Can you work these out from the model? Positions are in its coordinate system, mm. A direction names the side the tool comes from. Coordinates: 2 decimals unless noted, no trailing zeros. Loops run counter-clockwise (first coordinate to the right, second up) from the corner with the lowest first, then second, coordinate; pieces in that order, holes last. Notation, with made-up numbers: (72.25, -19.5) -> (113.25, -19.5) arc R35 ccw to (113.25, 14.5) -> close; hole circle Ø3 at (-21.5, 37.5). An arc over 180 degrees is marked (long way). Use one line per item in the form item = value. Start each with the question number.
(1) Imagine slicing it at A-A (x = 15). List the corners of the cut face in (y, z) for me, plus the area to 3 significant figures.
(2) On a 3-axis mill with a long thin cutter (end or side, diameter ignored), from which of +Z, -Z, +X, -X, +Y, -Y can I reach the whole of each face in a straight line? I mean faces 1 (the flat face through (-7.095, -3.109, -0.096)), 2 (the cylindrical face through (19.388, -5.224, 0.003)). Say none if no direction works.
(3) Imagine slicing it at B-B (y = -2.5). List the corners of the cut face in (x, z) for me, plus the area to 3 significant figures.
(4) I need wall thicknesses on line 1 (Y direction, x = 13.5, z = 0.05); line 2 (Y direction, x = 16.5, z = 0.1); line 3 (Y direction, x = 17.5, z = 0.1). Which ranges of each line are inside material? Lowest first, please. Write a range as [from, to].
(5) Thinking about a two-plate mould opening in X: for faces 3 (the flat face through (8, -1, 0.19)), 4 (the flat face through (21.98, -5.36, 0)), 5 (the cylindrical face through (17.016, -2.473, 0.003)), which applies, released by +X, released by -X, zero draft, split by the parting line, or undercut?
(6) Imagine slicing it at C-C (x = 3.5). List the corners of the cut face in (y, z) for me (3 decimals).
(7) Imagine slicing it at D-D (x = -12). List the corners of the cut face in (y, z) for me, plus the area to 3 significant figures.
```python
from build123d import *

# Parameters (mm, degrees)
BOSS_EXTRU_1_DEPTH           = 0.19
ENL_V_MAT_EXTRU_1_DEPTH      = 24.560167769
CONG_1_R                     = 0.25
ENL_V_MAT_EXTRU_2_DEPTH      = 21.94767488
ENL_V_MAT_EXTRU_2_DEPTH_BACK = 21.94767488


with BuildPart() as part:
    # Esquisse1 → Boss.-Extru.1 (new, symmetric)
    with BuildSketch(Plane.XY):
        with BuildLine():
            Line((-17.183394089, -0.900543525), (0, 0))
            Line((0, 0), (20, 0))
            Line((20, 0), (22.816605911, -4.878504542))
            Line((22.816605911, -4.878504542), (21.116605911, -5.86))
            ThreePointArc((21.116605911, -5.86), (19.362950472, -5.217969417), (17.508226773, -5))
            Line((17.508226773, -5), (4.724985048, -5))
            ThreePointArc((4.724985048, -5), (2.870261349, -5.217969417), (1.116605911, -5.86))
            Line((1.116605911, -5.86), (-17.183394089, -0.900543525))
        make_face()
    extrude(amount=BOSS_EXTRU_1_DEPTH, both=True)

    # Esquisse2 → Enlèv. mat.-Extru.1 (cut, through all)
    with BuildSketch(Plane.XY.offset(0.19)):
        with BuildLine():
            Line((-0.983394089, -1.85), (0.016605911, -1.85))
            Line((0.016605911, -1.85), (0.016605911, -1.675))
            Line((0.016605911, -1.675), (7.016605911, -1.675))
            Line((7.016605911, -1.675), (7.016605911, -1.25))
            Line((7.016605911, -1.25), (15.766605911, -1.25))
            ThreePointArc((15.766605911, -1.25), (17.016605911, -2.5), (15.766605911, -3.75))
            Line((15.766605911, -3.75), (7.016605911, -3.75))
            Line((7.016605911, -3.75), (7.016605911, -3.325))
            Line((7.016605911, -3.325), (0.016605911, -3.325))
            Line((0.016605911, -3.325), (0.016605911, -3.15))
            Line((0.016605911, -3.15), (-0.983394089, -3.15))
            Line((-0.983394089, -3.15), (-0.983394089, -1.85))
        make_face()
    extrude(amount=-ENL_V_MAT_EXTRU_1_DEPTH, mode=Mode.SUBTRACT)

    # Congé1
    # the kernel refuses this fillet: 0.25 mm, written as the material it adds along each edge
    with BuildSketch(Plane(origin=(7.016605911, -3.75, 0.19), x_dir=(0, 1, 0), z_dir=(0, 0, -1))) as cong_1_piece_1:
        with BuildLine():
            CenterArc((CONG_1_R, CONG_1_R), CONG_1_R, 180, 90)
            Line((0, CONG_1_R), (-CONG_1_R * 0.02, CONG_1_R))
            Line((-CONG_1_R * 0.02, CONG_1_R), (-CONG_1_R * 0.02, -CONG_1_R * 0.02))
            Line((-CONG_1_R * 0.02, -CONG_1_R * 0.02), (CONG_1_R, -CONG_1_R * 0.02))
            Line((CONG_1_R, -CONG_1_R * 0.02), (CONG_1_R, 0))
        make_face()
    extrude(amount=0.38)
    with BuildSketch(Plane(origin=(7.016605911, -1.25, 0.19), x_dir=(0, -1, 0), z_dir=(0, 0, -1)), Plane(origin=(-0.983394089, -3.15, 0.19), x_dir=(1, 0, 0), z_dir=(0, 0, -1)), Plane(origin=(-0.983394089, -1.85, 0.19), x_dir=(0, -1, 0), z_dir=(0, 0, -1))) as cong_1_piece_2:
        with BuildLine():
            CenterArc((CONG_1_R, -CONG_1_R), CONG_1_R, 90, 90)
            Line((0, -CONG_1_R), (-CONG_1_R * 0.02, -CONG_1_R))
            Line((-CONG_1_R * 0.02, -CONG_1_R), (-CONG_1_R * 0.02, CONG_1_R * 0.02))
            Line((-CONG_1_R * 0.02, CONG_1_R * 0.02), (CONG_1_R, CONG_1_R * 0.02))
            Line((CONG_1_R, CONG_1_R * 0.02), (CONG_1_R, 0))
        make_face()
    extrude(amount=0.38)
    with BuildSketch(Plane(origin=(0.016605911, -3.325, 0.19), x_dir=(1, 0, 0), z_dir=(0, 0, -1))) as cong_1_piece_3:
        with BuildLine():
            CenterArc((0.2384848, -0.25), CONG_1_R, 90, 72.542396876)
            Line((0, -0.175), (-0.004769696, -0.1735))
            ThreePointArc((-0.004769696, -0.1735), (-0.005, -0.0875), (-0.005, 0))
            Line((-0.005, 0), (0, 0.005))
            Line((0, 0.005), (0.2384848, 0.005))
            Line((0.2384848, 0.005), (0.2384848, 0))
        make_face()
    extrude(amount=0.38)
    with BuildSketch(Plane(origin=(0.016605911, -1.675, 0.19), x_dir=(0, -1, 0), z_dir=(0, 0, -1))) as cong_1_piece_4:
        with BuildLine():
            CenterArc((0.25, -0.2384848), CONG_1_R, 107.457603124, 72.542396876)
            Line((0, -0.2384848), (-0.005, -0.2384848))
            Line((-0.005, -0.2384848), (-0.005, 0))
            Line((-0.005, 0), (0, 0.005))
            ThreePointArc((0, 0.005), (0.0875, 0.005), (0.1735, 0.004769696))
            Line((0.1735, 0.004769696), (0.175, 0))
        make_face()
    extrude(amount=0.38)

    # Esquisse3 → Enlèv. mat.-Extru.2 (cut, two sides: drawn at the far end of the back side and taken through both)
    with BuildSketch(Plane(origin=(2.519658127, -0.682848897, 0), x_dir=(0, 0, 1), z_dir=(-0.9651836866427717, 0.26157303194073345, 0)).offset(-ENL_V_MAT_EXTRU_2_DEPTH_BACK)):
        Polygon((0, -5.36390241), (0.19, -4.36390241), (0.19, -5.53890241), (-0.19, -5.53890241), (-0.19, -4.36390241), align=None)
    extrude(amount=ENL_V_MAT_EXTRU_2_DEPTH + ENL_V_MAT_EXTRU_2_DEPTH_BACK, mode=Mode.SUBTRACT)


solid = part.part
```
Worked out:
q1.outline = (-5, -0.19) -> (-3.75, -0.19) -> (-3.75, 0.19) -> (-5, 0.19) -> close; (-1.25, -0.19) -> (0, -0.19) -> (0, 0.19) -> (-1.25, 0.19) -> close
q1.area = 0.950 mm2
q2.face_1 = -Z, -X, -Y
q2.face_2 = +Z, -Z, -Y
q3.outline = (-11.28, 0) -> (-7.46, -0.19) -> (-0.98, -0.19) -> (-0.98, 0.19) -> (-7.46, 0.19) -> close; (17.02, -0.19) -> (21.44, -0.19) -> (21.44, 0.19) -> (17.02, 0.19) -> close
q3.area = 4.87 mm2
q4.line_1 = [-5, -3.75], [-1.25, 0]
q4.line_2 = [-5, -3.51], [-1.49, 0]
q4.line_3 = [-5, 0]
q5.face_3 = zero draft
q5.face_4 = released by +X
q5.face_5 = undercut
q6.outline = (-5.094, -0.19) -> (-3.325, -0.19) -> (-3.325, 0.19) -> (-5.094, 0.19) -> close; (-1.675, -0.19) -> (0, -0.19) -> (0, 0.19) -> (-1.675, 0.19) -> close
q7.outline = (-2.31, 0) -> (-1.27, -0.19) -> (-0.63, -0.19) -> (-0.63, 0.19) -> (-1.27, 0.19) -> close
q7.area = 0.440 mm2
